Here's how the part is built. I have some questions about the finished solid (model axes, mm). A direction names the side the tool comes from. Coordinates: 2 decimals unless noted, no trailing zeros. Order: outer loops, then holes, each group sorted by start corner. A loop starts at its lowest first (then second) coordinate and runs counter-clockwise, first axis right, second up. Notation, with made-up numbers: (-12, 17) - (40, 17) arc R20 cw to (40, 52) - close; hole circle Ø3 at (58, 83.5). An arc over 180 degrees is marked (long way). Answer in a Markdown table with one row per item. Add a question column.
Item 1: If I drill on line 1 along X through (y, z) = (-5.45, 7.1); line 2 along Y through (x, z) = (5, -8.5); line 3 along X through (y, z) = (0.75, 7.25), over which ranges is the centre line in solid material (lowest first)? Write a range as from..to.
Item 2: I want a section at B-B (x = -5). Please give me the cut outline in (y, z).
Item 3: Will these pins go through, and if not, where does the flat tip stop? pin 1 Ø6 at (x, y) = (-4, -1) entering from +Z; pin 2 Ø2 at (y, z) = (1, 5.5) entering from +X; pin 3 Ø3 at (x, z) = (10, 5.5) entering from +Y.
Item 4: Thinking about a two-plate mould opening in Z: for faces 1 (the cylindrical face through (15.76, -5.33, 4.33)), 2 (the flat face through (13.2, -3.85, 7.1)), 3 (the cylindrical face through (-6.774, -5.329, 8.023)), 4 (the flat face through (-5, -5, 10.1)), which applies, +Z half, -Z half, draft (parallel to the pull), parting line (faces both ways), or undercut?
Item 5: On a 3-axis mill with a long thin cutter (end or side, diameter ignored), from which of +Z, -Z, +X, -X, +Y, -Y can I reach the whole of each face in a straight line? I mean faces 5 (the flat face through (11, -5, 4.1)), 6 (the flat face through (-7.3, -3.85, 7.1)), 7 (the flat face through (-5, -5, 4.1)), 8 (the flat face through (3, 2.5, -6)). Say none if no direction works.
Item 6: I want a section at C-C (z = 7.1). Please give me the cut outline in (x, y).
Item 7: I want a section at D-D (x = 3.5). Please give me the cut outline in (y, z), plus the area to 3 significant figures.
Item 8: I want a section at A-A (z = -4.5). Please give me the cut outline in (x, y), plus the area to 3 significant figures.
```python
from build123d import *

# Parameters (mm, degrees)
BOSS_EXTRUDE1_DEPTH      = 6
BOSS_EXTRUDE2_DEPTH      = 10
BOSS_EXTRUDE2_DEPTH_BACK = 16
SKETCH2_W                = 6
SKETCH2_H                = 3
SKETCH3_R                = 2
CUT_EXTRUDE1_DEPTH       = 10
FILLET1_R                = 0.8


with BuildPart() as part:
    # Sketch1 → Boss-Extrude1 (new body)
    with BuildSketch(Plane(origin=(0, 0, 0), x_dir=(0, 0, -1), z_dir=(1, 0, 0))):
        Polygon((11.1, 6.85), (-11.1, 6.85), (-11.1, -6.85), (11.1, -6.85), (11.1, -2.5), (1.1, -2.5), (1.1, 2.5), (11.1, 2.5), align=None)
    extrude(amount=BOSS_EXTRUDE1_DEPTH)

    # Sketch2 → Boss-Extrude2 (add, two sides: drawn at the far end of the back side and taken through both)
    with BuildSketch(Plane(origin=(6, 0, 0), x_dir=(0, 0, -1), z_dir=(1, 0, 0)).offset(-BOSS_EXTRUDE2_DEPTH_BACK)):
        with Locations((-7.1, -5.35)):
            Rectangle(SKETCH2_W, SKETCH2_H)
    extrude(amount=BOSS_EXTRUDE2_DEPTH + BOSS_EXTRUDE2_DEPTH_BACK)

    # Sketch3 → Cut-Extrude1 (cut)
    with BuildSketch(Plane(origin=(0, -3.85, 0), x_dir=(1, 0, 0), z_dir=(0, 1, 0))):
        with Locations(Location((11, -7.1, 0), (0, 0, 270))):
            Circle(SKETCH3_R)
        with Locations(Location((-5, -7.1, 0), (0, 0, 270))):
            Circle(SKETCH3_R)
    extrude(amount=-CUT_EXTRUDE1_DEPTH, mode=Mode.SUBTRACT)

    # Fillet1
    fillet1_edges = [part.edges().sort_by_distance(p)[0] for p in [
        (-10, -5.35, 4.1),
        (-10, -5.35, 10.1),
        (16, -5.35, 4.1),
        (16, -5.35, 10.1),
    ]]
    fillet(fillet1_edges, radius=FILLET1_R)


solid = part.part
```
Values follow:
| question | item | result |
|---|---|---|
| 1 | line 1 | x = -10..-7, -3..9, 13..16 |
| 1 | line 2 | y = -6.85..-2.5, 2.5..6.85 |
| 1 | line 3 | x = 0..6 |
| 2 | outline | (-6.85, 4.1) - (-3.85, 4.1) - (-3.85, 5.1) - (-6.85, 5.1) - close; (-6.85, 9.1) - (-3.85, 9.1) - (-3.85, 10.1) - (-6.85, 10.1) - close |
| 3 | pin 1 | stops at z = 10.1 |
| 3 | pin 2 | stops at x = 6 |
| 3 | pin 3 | stops at y = -3.85 |
| 4 | face 1 | -Z half |
| 4 | face 2 | draft |
| 4 | face 3 | undercut |
| 4 | face 4 | +Z half |
| 5 | face 5 | -Z, +X, +Y, -Y |
| 5 | face 6 | +Z, -Z, -X, +Y |
| 5 | face 7 | -Z, -X, +Y, -Y |
| 5 | face 8 | -Z, +X, -X |
| 6 | outline | (-10, -6.85) - (-7, -6.85) - (-7, -3.85) - (-10, -3.85) - close; (-3, -6.85) - (9, -6.85) - (9, -3.85) - (6, -3.85) - (6, 6.85) - (0, 6.85) - (0, -3.85) - (-3, -3.85) - close; (13, -6.85) - (16, -6.85) - (16, -3.85) - (13, -3.85) - close |
| 7 | outline | (-6.85, -11.1) - (-2.5, -11.1) - (-2.5, -1.1) - (2.5, -1.1) - (2.5, -11.1) - (6.85, -11.1) - (6.85, 11.1) - (-6.85, 11.1) - close |
| 7 | area | 254 mm^2 |
| 8 | outline | (0, -6.85) - (6, -6.85) - (6, -2.5) - (0, -2.5) - close; (0, 2.5) - (6, 2.5) - (6, 6.85) - (0, 6.85) - close |
| 8 | area | 52.2 mm^2 |
